from build123d import *

# Parameters (mm, degrees)
F0_W     = 19.05
F0_H     = 3.175
F1_DEPTH = 38.1
F2_R     = 1.984375
F3_DEPTH = 3.175


with BuildPart() as f1:
    # F0 (on Top) → F1 (new body, symmetric)
    with BuildSketch(Plane.XY):
        Rectangle(F0_W, F0_H)
    extrude(amount=F1_DEPTH, both=True)

    # F2 (on face) → F3 (cut, through all)
    with BuildSketch(Plane.XZ.offset(1.5875)):
        with Locations((3.175, 25.4)):
            Circle(F2_R)
        with Locations((-3.175, 25.4)):
            Circle(F2_R)
        with Locations((3.175, 6.35)):
            Circle(F2_R)
        with Locations((-3.175, 6.35)):
            Circle(F2_R)
    extrude(amount=-F3_DEPTH, mode=Mode.SUBTRACT)


solid = f1.part
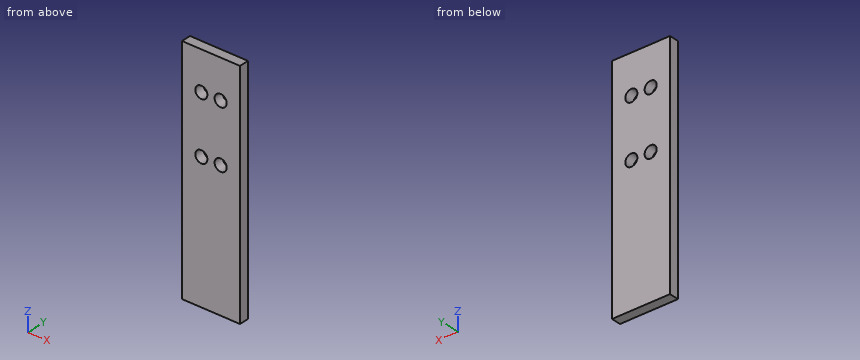
The listing builds one solid part. Answer for the finished solid, in the listing's coordinates (mm). Give positions to 0.01 mm unless a question says otherwise; leave off trailing zeros. Order: outer loops, then holes, each group sorted by start corner. A loop starts at its lowest first (then second) coordinate and runs counter-clockwise, first axis right, second up. Notation, with made-up numbers: (16, -0.5) - (66, -0.5) arc R16 cw to (66, 15.5) - close; hole circle Ø8 at (6.25, 85). An arc over 180 degrees is marked (long way). Use one line per item in the form item = value.
1) Consider probe 1 along Z at (x, y) = (-3.5, -1.3); probe 2 along Z at (x, y) = (4.5, -0.45). Determine where each line is inside the solid, lowest interval first. Write a range as [from, to].
Verdict:
probe_1 = [-38.1, 4.39], [8.31, 23.44], [27.36, 38.1]
probe_2 = [-38.1, 4.87], [7.83, 23.92], [26.88, 38.1]
2) This flat-tipped pin is pushed along its axis until it touches: pin 1 (5 mm diameter, centred on x = 3.175, z = 25.4, fed in from +Y). Where does it stop, or does it pass through?
Verdict:
pin_1 = 1.59
3) Find section B-B on z = 6.35. Determine the outline of the cut face in (x, y) (1 decimal), and give its area (3 significant figures).
Verdict:
outline = (-9.5, -1.6) - (-5.2, -1.6) - (-5.2, 1.6) - (-9.5, 1.6) - close; (-1.2, -1.6) - (1.2, -1.6) - (1.2, 1.6) - (-1.2, 1.6) - close; (5.2, -1.6) - (9.5, -1.6) - (9.5, 1.6) - (5.2, 1.6) - close
area = 35.3 mm^2
4) Find section A-A on y = 1.05. Determine the outline of the cut face in (x, z) (3 decimals).
Verdict:
outline = (-9.525, -38.1) - (9.525, -38.1) - (9.525, 38.1) - (-9.525, 38.1) - close; hole circle Ø3.969 at (-3.175, 6.35); hole circle Ø3.969 at (-3.175, 25.4); hole circle Ø3.969 at (3.175, 6.35); hole circle Ø3.969 at (3.175, 25.4)
5) Find section C-C on x = -3.25. Determine the outline of the cut face in (y, z).
Verdict:
outline = (-1.59, -38.1) - (1.59, -38.1) - (1.59, 4.37) - (-1.59, 4.37) - close; (-1.59, 8.33) - (1.59, 8.33) - (1.59, 23.42) - (-1.59, 23.42) - close; (-1.59, 27.38) - (1.59, 27.38) - (1.59, 38.1) - (-1.59, 38.1) - close
